Could you check a few things on this model? Use its own coordinates, in mm. A direction names the side the tool comes from. Coordinates: 2 decimals unless noted, no trailing zeros. Loops run counter-clockwise (first coordinate to the right, second up) from the corner with the lowest first, then second, coordinate; pieces in that order, holes last. Notation, with made-up numbers: (56, 30.25) - (68, 30.25) arc R3 cw to (68, 35.25) - close; hole circle Ø10 at (31, -7). An arc over 180 degrees is marked (long way). Use CSV: the item, a comma, the result in double quotes.
Autodesk Inventor part; units mm, degrees
ref_plane "YZ Plane" through (0, 0, 0) normal (1, 0, 0) x (0, 1, 0)
ref_plane "XZ Plane" through (0, 0, 0) normal (0, 1, 0) x (-1, 0, 0)
ref_plane "XY Plane" through (0, 0, 0) normal (0, 0, 1) x (1, 0, 0)
sketch "Sketch1" plane through (0, 0, 0) normal (0, 0, 1) x (1, 0, 0)
  line L0 (-10.4228, -30) -> (-12.9228, -30)
  line L1 (-12.9228, -30) -> (-12.9228, -27)
  line L2 (-12.9228, -27) -> (-10.4228, -27)
  line L3 (-10.4228, -27) -> (-10.4228, -30)
  line L4 (-10.4228, -30) -> (-10.4228, -55)
  line L5 (-10.4228, -55) -> (-11.9228, -55)
  line L6 (-11.9228, -55) -> (-11.9228, -30)
  point P0 (0, 0)
  dimension "d0" = 2.5
  dimension "d1" = 3
  dimension "d3" = 1.5
  dimension "d16" = 25
revolve "Revolution1" add sketch "Sketch1" angle 360 about axis through (-10.4228, -30, 0) along (0, -1, 0)
chamfer "Chamfer1" distance 0.2 angle 45 1 edges at (-7.9228, -27, 0)
sketch "Boceto2" plane through (-10.4228, -27, 0) normal (0, 1, 0) x (1, 0, 0)
  line L0 (0.5669, -0.6547) -> (-0.2835, -0.8183)
  line L1 (-0.2835, -0.8183) -> (-0.8504, -0.1636)
  line L2 (-0.8504, -0.1636) -> (-0.5669, 0.6547)
  line L3 (-0.5669, 0.6547) -> (0.2835, 0.8183)
  line L4 (0.2835, 0.8183) -> (0.8504, 0.1636)
  line L5 (0.8504, 0.1636) -> (0.5669, -0.6547)
  point P0 (10.4228, 0)
  point P1 (0, 0)
  dimension "d11" = 1.5
extrude "Extrusión1" cut sketch "Boceto2" against normal blind 2
fillet "Fillet1" radius 0.1 1 edges at (-8.9228, -30, 0)
chamfer "Chamfer3" distance 0.2 angle 45 1 edges at (-8.9228, -55, 0)
chamfer "Chamfer4" distance 0.08 angle 45 1 edges at (-7.9228, -30, 0)
thread "Thread3"
properties part number "Tornillo Allen cabeza cilindrica M3x20mm"
(1) Suppose I cut it at A-A (y = -38.5). Write out the boundary of the cut face in (x, z).
Computed:
outline,"circle Ø3 at (-10.42, 0)"
(2) Thinking about a two-plate mould opening in Y: for faces 4 (the face through (-10, -55, 0)), 5 (the face through (-10, -27, -1)), 6 (the face through (-11.81, -42.28, -0.57)), which applies, +Y half, -Y half, draft (parallel to the pull), parting line (faces both ways), or undercut?
Computed:
face 4,"-Y half"
face 5,"+Y half"
face 6,"draft"
(3) Will these pins go through, and if not, where does the flat tip stop? pin 1 (1.8 mm diameter, centred on x = -10.5, z = 0.5, fed in from +Y); pin 2 (2 mm diameter, centred on y = -39.5, z = 0.5, fed in from -X).
Computed:
pin 1,"stops at y = -27"
pin 2,"stops at x = -11.92"
(4) Which directions (+Z, -Z, +X, -X, +Y, -Y) give clear straight access to the entire face, cutting with the end or side of a thin tool? Please do faces 1 (the face through (-10.57, -27.986, -0.735)), 2 (the face through (-12.807, -28.541, 0.751)), 3 (the face through (-11, -30, 2)).
Computed:
face 1,"+Y"
face 2,"+Y, -Y"
face 3,"-Y"
(5) Please list where these lines run through material, in increasing order: line 1 (Y direction, x = -10.2, z = 1.55); line 2 (Z direction, x = -10.5, y = -33.25); line 3 (X direction, y = -31.5, z = 0.05).
Computed:
line 1,"y = -30.01 to -27"
line 2,"z = -1.5 to 1.5"
line 3,"x = -11.92 to -8.92"
